Check sheet for the modelled part. Datum: model origin and axes. Units: mm. Give positions to 0.01 mm unless a question says otherwise; leave off trailing zeros. Order: outer loops, then holes, each group sorted by start corner. A loop starts at its lowest first (then second) coordinate and runs counter-clockwise, first axis right, second up. Notation, with made-up numbers: (-4.5, 52) -> (54.5, 52) arc R37 ccw to (54.5, 88) -> close; hole circle Ø3 at (-29, -38). An arc over 180 degrees is marked (long way). Write each question's results on one line, items separated by ' | '.
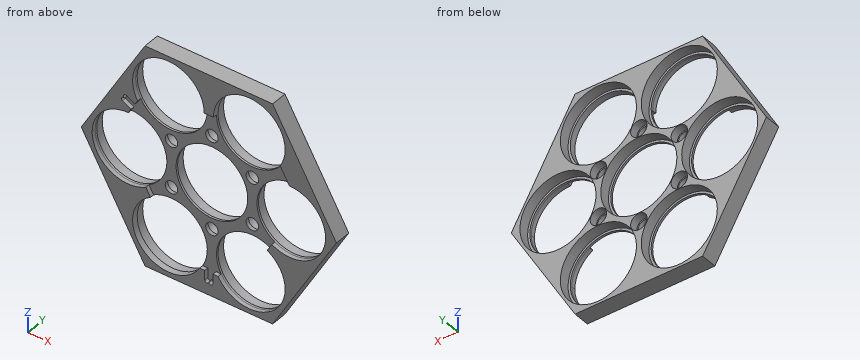
from build123d import *

# Parameters (mm, degrees)
SKETCH1_R                    = 17.5
BOSS_EXTRUDE1_DEPTH          = 1
SKETCH2_R                    = 18.575
BOSS_EXTRUDE2_DEPTH          = 5
CUT_EXTRUDE1_DEPTH           = 83.640310894
CUT_EXTRUDE1_DEPTH_BACK      = 4
SKETCH3_R                    = 4
SKETCH3_2_R                  = 4
CUT_EXTRUDE2_DEPTH           = 83.640310894
CUT_EXTRUDE2_DRAFT           = -9
CUT_EXTRUDE2_PROFILE_2_DEPTH = 83.640310894
CUT_EXTRUDE2_PROFILE_2_DRAFT = -9
CUT_EXTRUDE2_PROFILE_3_DEPTH = 83.640310894
CUT_EXTRUDE2_PROFILE_3_DRAFT = -9
CUT_EXTRUDE2_PROFILE_4_DEPTH = 83.640310894
CUT_EXTRUDE2_PROFILE_4_DRAFT = -9
CUT_EXTRUDE2_PROFILE_5_DEPTH = 83.640310894
CUT_EXTRUDE2_PROFILE_5_DRAFT = -9
CUT_EXTRUDE2_PROFILE_6_DEPTH = 83.640310894
CUT_EXTRUDE2_PROFILE_6_DRAFT = -9
BOSS_EXTRUDE3_START          = 2
BOSS_EXTRUDE3_DEPTH          = 2
CUT_EXTRUDE5_DEPTH           = 2


with BuildPart() as part:
    # Sketch1 → Boss-Extrude1 (new body)
    with BuildSketch(Plane(origin=(0, 0, 0), x_dir=(1, 0, 0), z_dir=(0, 1, 0))):
        Polygon((-31.152667816, -53.958003449), (31.152667816, -53.958003449), (62.305335633, 0), (31.152667816, 53.958003449), (-31.152667816, 53.958003449), (-62.305335633, 0), align=None)
        with Locations(Location((-39.5, 0, 0), (0, 0, 270))):
            Circle(SKETCH1_R, mode=Mode.SUBTRACT)
        with Locations(Location((-19.75, -34.208003449, 0), (0, 0, 270))):
            Circle(SKETCH1_R, mode=Mode.SUBTRACT)
        with Locations(Location((19.75, -34.208003449, 0), (0, 0, 270))):
            Circle(SKETCH1_R, mode=Mode.SUBTRACT)
        with Locations(Location((39.5, 0, 0), (0, 0, 270))):
            Circle(SKETCH1_R, mode=Mode.SUBTRACT)
        with Locations(Location((19.75, 34.208003449, 0), (0, 0, 270))):
            Circle(SKETCH1_R, mode=Mode.SUBTRACT)
        with Locations(Location((-19.75, 34.208003449, 0), (0, 0, 270))):
            Circle(SKETCH1_R, mode=Mode.SUBTRACT)
        with Locations(Location((0, 0, 0), (0, 0, 270))):
            Circle(SKETCH1_R, mode=Mode.SUBTRACT)
    extrude(amount=BOSS_EXTRUDE1_DEPTH)

    # Sketch2 → Boss-Extrude2 (add)
    with BuildSketch(Plane(origin=(0, 1, 0), x_dir=(1, 0, 0), z_dir=(0, 1, 0))):
        Polygon((62.305335633, 0), (31.152667816, 53.958003449), (-31.152667816, 53.958003449), (-62.305335633, 0), (-31.152667816, -53.958003449), (31.152667816, -53.958003449), align=None)
        with Locations(Location((-39.5, 0, 0), (0, 0, 270))):
            Circle(SKETCH2_R, mode=Mode.SUBTRACT)
        with Locations(Location((-19.75, 34.208003449, 0), (0, 0, 270))):
            Circle(SKETCH2_R, mode=Mode.SUBTRACT)
        with Locations(Location((19.75, 34.208003449, 0), (0, 0, 270))):
            Circle(SKETCH2_R, mode=Mode.SUBTRACT)
        with Locations(Location((0, 0, 0), (0, 0, 270))):
            Circle(SKETCH2_R, mode=Mode.SUBTRACT)
        with Locations(Location((39.5, 0, 0), (0, 0, 270))):
            Circle(SKETCH2_R, mode=Mode.SUBTRACT)
        with Locations(Location((19.75, -34.208003449, 0), (0, 0, 270))):
            Circle(SKETCH2_R, mode=Mode.SUBTRACT)
        with Locations(Location((-19.75, -34.208003449, 0), (0, 0, 270))):
            Circle(SKETCH2_R, mode=Mode.SUBTRACT)
    extrude(amount=BOSS_EXTRUDE2_DEPTH)

    # Sketch3 → Cut-Extrude1 (cut, two sides: drawn at the far end of the back side and taken through both)
    with BuildSketch(Plane(origin=(0, 6, 0), x_dir=(1, 0, 0), z_dir=(0, 1, 0)).offset(-CUT_EXTRUDE1_DEPTH_BACK)):
        with Locations(Location((-19.75, 11.402667816, 0), (0, 0, 90))):
            Circle(SKETCH3_R)
        with Locations(Location((19.75, 11.402667816, 0), (0, 0, 90))):
            Circle(SKETCH3_R)
        with Locations(Location((0, -22.805335633, 0), (0, 0, 90))):
            Circle(SKETCH3_R)
        with Locations(Location((-19.75, -11.402667816, 0), (0, 0, 90))):
            Circle(SKETCH3_R)
        with Locations(Location((19.75, -11.402667816, 0), (0, 0, 90))):
            Circle(SKETCH3_R)
        with Locations(Location((0, 22.805335633, 0), (0, 0, 90))):
            Circle(SKETCH3_R)
    extrude(amount=CUT_EXTRUDE1_DEPTH + CUT_EXTRUDE1_DEPTH_BACK, mode=Mode.SUBTRACT)


with BuildPart() as cut_extrude2_tool:
    # Sketch3<2> → Cut-Extrude2 (with draft: the straight prism first)
    with BuildSketch(Plane(origin=(0, 6, 0), x_dir=(1, 0, 0), z_dir=(0, 1, 0))):
        with Locations(Location((-19.75, 11.402667816, 0), (0, 0, 90))):
            Circle(SKETCH3_2_R)
    extrude(amount=-CUT_EXTRUDE2_DEPTH)
    # Cut-Extrude2: the draft: its side faces are tilted about the plane it starts from
    cut_extrude2_sides = [cut_extrude2_tool.faces().sort_by_distance(p)[0] for p in [
        (-19.75, -35.820155447, -7.402667816),
    ]]
    draft(cut_extrude2_sides, Plane(origin=(0, 6, 0), x_dir=(1, 0, 0), z_dir=(0, 1, 0)), CUT_EXTRUDE2_DRAFT)


with BuildPart() as part_1:
    add(part.part)

    # Cut-Extrude2: cut by cut_extrude2_tool
    add(cut_extrude2_tool.part, mode=Mode.SUBTRACT)


with BuildPart() as cut_extrude2_profile_2_tool:
    # Sketch3<2> → Cut-Extrude2 profile 2 (with draft: the straight prism first)
    with BuildSketch(Plane(origin=(0, 6, 0), x_dir=(1, 0, 0), z_dir=(0, 1, 0))):
        with Locations(Location((19.75, 11.402667816, 0), (0, 0, 90))):
            Circle(SKETCH3_2_R)
    extrude(amount=-CUT_EXTRUDE2_PROFILE_2_DEPTH)
    # Cut-Extrude2 profile 2: the draft: its side faces are tilted about the plane it starts from
    cut_extrude2_profile_2_sides = [cut_extrude2_profile_2_tool.faces().sort_by_distance(p)[0] for p in [
        (19.75, -35.820155447, -7.402667816),
    ]]
    draft(cut_extrude2_profile_2_sides, Plane(origin=(0, 6, 0), x_dir=(1, 0, 0), z_dir=(0, 1, 0)), CUT_EXTRUDE2_PROFILE_2_DRAFT)


with BuildPart() as part_2:
    add(part_1.part)

    # Cut-Extrude2 profile 2: cut by cut_extrude2_profile_2_tool
    add(cut_extrude2_profile_2_tool.part, mode=Mode.SUBTRACT)


with BuildPart() as cut_extrude2_profile_3_tool:
    # Sketch3<2> → Cut-Extrude2 profile 3 (with draft: the straight prism first)
    with BuildSketch(Plane(origin=(0, 6, 0), x_dir=(1, 0, 0), z_dir=(0, 1, 0))):
        with Locations(Location((0, -22.805335633, 0), (0, 0, 90))):
            Circle(SKETCH3_2_R)
    extrude(amount=-CUT_EXTRUDE2_PROFILE_3_DEPTH)
    # Cut-Extrude2 profile 3: the draft: its side faces are tilted about the plane it starts from
    cut_extrude2_profile_3_sides = [cut_extrude2_profile_3_tool.faces().sort_by_distance(p)[0] for p in [
        (0, -35.820155447, 26.805335633),
    ]]
    draft(cut_extrude2_profile_3_sides, Plane(origin=(0, 6, 0), x_dir=(1, 0, 0), z_dir=(0, 1, 0)), CUT_EXTRUDE2_PROFILE_3_DRAFT)


with BuildPart() as part_3:
    add(part_2.part)

    # Cut-Extrude2 profile 3: cut by cut_extrude2_profile_3_tool
    add(cut_extrude2_profile_3_tool.part, mode=Mode.SUBTRACT)


with BuildPart() as cut_extrude2_profile_4_tool:
    # Sketch3<2> → Cut-Extrude2 profile 4 (with draft: the straight prism first)
    with BuildSketch(Plane(origin=(0, 6, 0), x_dir=(1, 0, 0), z_dir=(0, 1, 0))):
        with Locations(Location((-19.75, -11.402667816, 0), (0, 0, 90))):
            Circle(SKETCH3_2_R)
    extrude(amount=-CUT_EXTRUDE2_PROFILE_4_DEPTH)
    # Cut-Extrude2 profile 4: the draft: its side faces are tilted about the plane it starts from
    cut_extrude2_profile_4_sides = [cut_extrude2_profile_4_tool.faces().sort_by_distance(p)[0] for p in [
        (-19.75, -35.820155447, 15.402667816),
    ]]
    draft(cut_extrude2_profile_4_sides, Plane(origin=(0, 6, 0), x_dir=(1, 0, 0), z_dir=(0, 1, 0)), CUT_EXTRUDE2_PROFILE_4_DRAFT)


with BuildPart() as part_4:
    add(part_3.part)

    # Cut-Extrude2 profile 4: cut by cut_extrude2_profile_4_tool
    add(cut_extrude2_profile_4_tool.part, mode=Mode.SUBTRACT)


with BuildPart() as cut_extrude2_profile_5_tool:
    # Sketch3<2> → Cut-Extrude2 profile 5 (with draft: the straight prism first)
    with BuildSketch(Plane(origin=(0, 6, 0), x_dir=(1, 0, 0), z_dir=(0, 1, 0))):
        with Locations(Location((19.75, -11.402667816, 0), (0, 0, 90))):
            Circle(SKETCH3_2_R)
    extrude(amount=-CUT_EXTRUDE2_PROFILE_5_DEPTH)
    # Cut-Extrude2 profile 5: the draft: its side faces are tilted about the plane it starts from
    cut_extrude2_profile_5_sides = [cut_extrude2_profile_5_tool.faces().sort_by_distance(p)[0] for p in [
        (19.75, -35.820155447, 15.402667816),
    ]]
    draft(cut_extrude2_profile_5_sides, Plane(origin=(0, 6, 0), x_dir=(1, 0, 0), z_dir=(0, 1, 0)), CUT_EXTRUDE2_PROFILE_5_DRAFT)


with BuildPart() as part_5:
    add(part_4.part)

    # Cut-Extrude2 profile 5: cut by cut_extrude2_profile_5_tool
    add(cut_extrude2_profile_5_tool.part, mode=Mode.SUBTRACT)


with BuildPart() as cut_extrude2_profile_6_tool:
    # Sketch3<2> → Cut-Extrude2 profile 6 (with draft: the straight prism first)
    with BuildSketch(Plane(origin=(0, 6, 0), x_dir=(1, 0, 0), z_dir=(0, 1, 0))):
        with Locations(Location((0, 22.805335633, 0), (0, 0, 90))):
            Circle(SKETCH3_2_R)
    extrude(amount=-CUT_EXTRUDE2_PROFILE_6_DEPTH)
    # Cut-Extrude2 profile 6: the draft: its side faces are tilted about the plane it starts from
    cut_extrude2_profile_6_sides = [cut_extrude2_profile_6_tool.faces().sort_by_distance(p)[0] for p in [
        (0, -35.820155447, -18.805335633),
    ]]
    draft(cut_extrude2_profile_6_sides, Plane(origin=(0, 6, 0), x_dir=(1, 0, 0), z_dir=(0, 1, 0)), CUT_EXTRUDE2_PROFILE_6_DRAFT)


with BuildPart() as part_6:
    add(part_5.part)

    # Cut-Extrude2 profile 6: cut by cut_extrude2_profile_6_tool
    add(cut_extrude2_profile_6_tool.part, mode=Mode.SUBTRACT)

    # Sketch5 → Boss-Extrude3 (add)
    with BuildSketch(Plane.XZ.offset(BOSS_EXTRUDE3_START)):
        with BuildLine():
            Line((-31.152667816, 53.958003449), (-62.305335633, 0))
            Line((-62.305335633, 0), (-57, 0))
            ThreePointArc((-57, 0), (-51.812065653, 12.43635957), (-39.324224074, 17.499117201))
            Line((-39.324224074, 17.499117201), (-34.816792077, 25.306218432))
            ThreePointArc((-34.816792077, 25.306218432), (-24.364170491, 51.088744863), (-2.25, 34.208003449))
            Line((-2.25, 34.208003449), (2.25, 34.208003449))
            ThreePointArc((2.25, 34.208003449), (11, 49.363448016), (28.5, 49.363448016))
            Line((28.5, 49.363448016), (31.152667816, 53.958003449))
            Line((31.152667816, 53.958003449), (-31.152667816, 53.958003449))
        make_face()
        with BuildLine():
            Line((-57, 0), (-62.305335633, 0))
            Line((-62.305335633, 0), (-31.152667816, -53.958003449))
            Line((-31.152667816, -53.958003449), (31.152667816, -53.958003449))
            Line((31.152667816, -53.958003449), (28.5, -49.363448016))
            ThreePointArc((28.5, -49.363448016), (15.135829509, -51.088744863), (4.507431997, -42.805335633))
            Line((4.507431997, -42.805335633), (-4.507431997, -42.805335633))
            ThreePointArc((-4.507431997, -42.805335633), (-32.062065653, -46.644363019), (-28.5, -19.052558883))
            Line((-28.5, -19.052558883), (-30.75, -15.155444566))
            ThreePointArc((-30.75, -15.155444566), (-48.25, -15.155444566), (-57, 0))
        make_face()
        with BuildLine():
            Line((28.5, -49.363448016), (31.152667816, -53.958003449))
            Line((31.152667816, -53.958003449), (62.305335633, 0))
            Line((62.305335633, 0), (31.152667816, 53.958003449))
            Line((31.152667816, 53.958003449), (28.5, 49.363448016))
            ThreePointArc((28.5, 49.363448016), (34.905444566, 42.958003449), (37.25, 34.208003449))
            ThreePointArc((37.25, 34.208003449), (36.630741414, 29.593832958), (34.816792077, 25.306218432))
            Line((34.816792077, 25.306218432), (39.324224074, 17.499117201))
            ThreePointArc((39.324224074, 17.499117201), (51.812065653, 12.43635957), (57, 0))
            ThreePointArc((57, 0), (48.25, -15.155444566), (30.75, -15.155444566))
            Line((30.75, -15.155444566), (28.5, -19.052558883))
            ThreePointArc((28.5, -19.052558883), (34.905444566, -25.458003449), (37.25, -34.208003449))
            ThreePointArc((37.25, -34.208003449), (34.905444566, -42.958003449), (28.5, -49.363448016))
        make_face()
    extrude(amount=-BOSS_EXTRUDE3_DEPTH)

    # Sketch6 → Cut-Extrude5 (cut)
    with BuildSketch(Plane.XZ.offset(2)):
        with BuildLine():
            ThreePointArc((-2, -47.537386441), (-1, -48.537386441), (0, -47.537386441))
            ThreePointArc((0, -47.537386441), (1, -48.537386441), (2, -47.537386441))
            Line((2, -47.537386441), (2, -42.805335633))
            Line((2, -42.805335633), (-2, -42.805335633))
            Line((-2, -42.805335633), (-2, -47.537386441))
        make_face()
        with BuildLine():
            ThreePointArc((-40.168584287, 25.500744028), (-41.534609686, 25.134718633), (-41.168584305, 23.76869323))
            ThreePointArc((-41.168584305, 23.76869323), (-42.534609696, 23.402667808), (-42.168584287, 22.036642413))
            Line((-42.168584287, 22.036642413), (-38.070508076, 19.670617009))
            Line((-38.070508076, 19.670617009), (-36.070508076, 23.134718624))
            Line((-36.070508076, 23.134718624), (-40.168584287, 25.500744028))
        make_face()
    extrude(amount=-CUT_EXTRUDE5_DEPTH, mode=Mode.SUBTRACT)


solid = part_6.part
1. Section check C-C on x = -14. Record the cut outline in (y, z), then the cut area to 3 significant figures.
Verdict:
outline: (-2, -53.96) -> (6, -53.96) -> (6, -51.87) -> (1, -51.87) -> (1, -50.74) -> (-2, -50.74) -> close; (-2, 50.74) -> (1, 50.74) -> (1, 51.87) -> (6, 51.87) -> (6, 53.96) -> (-2, 53.96) -> close; (0, -17.68) -> (1, -17.68) -> (1, -16.55) -> (6, -16.55) -> (6, -12.21) -> (1, -12.21) -> (1, -10.5) -> (0, -10.5) -> close; (0, 10.5) -> (1, 10.5) -> (1, 12.21) -> (6, 12.21) -> (6, 16.55) -> (1, 16.55) -> (1, 17.68) -> (0, 17.68) -> close | area: 97.9 mm^2
2. Section check B-B on z = -30. Record the cut outline in (x, y).
Verdict:
outline: (-44.98, -2) -> (-36.74, -2) -> (-36.74, 1) -> (-37.84, 1) -> (-37.84, 6) -> (-44.98, 6) -> close; (-2.76, 0) -> (2.76, 0) -> (2.76, 1) -> (1.66, 1) -> (1.66, 6) -> (-1.66, 6) -> (-1.66, 1) -> (-2.76, 1) -> close; (36.74, -2) -> (44.98, -2) -> (44.98, 6) -> (37.84, 6) -> (37.84, 1) -> (36.74, 1) -> close
3. Material ranges on probe 1 along X at (y, z) = (0.7, 0); probe 2 along X at (y, z) = (5, 0) (3 decimals); probe 3 along X at (y, z) = (2.5, 31), recorded low to high. Write a range as from..to.
Verdict:
probe 1: x = -62.31..-57, -22..-17.5, 17.5..22, 57..62.31 | probe 2: x = -62.305..-58.075, -20.925..-18.575, 18.575..20.925, 58.075..62.305 | probe 3: x = -44.41..-38.05, -1.45..1.45, 38.05..44.41
4. Section check A-A on y = 4.75. Give the number of separate pieces and of enclosed holes in the cut face, then the cut area to 3 significant figures.
Verdict:
separate pieces: 1 | enclosed holes: 13 | area: 2,200 mm^2
5. Gauge pin test, flat ends, axial feed: pin 1 Ø1.5 at (y, z) = (4.5, -12) entering from -X; pin 2 Ø21 at (x, z) = (19.75, 34.21) entering from -Y; pin 3 Ø10.5 at (x, z) = (0, 22.81) entering from -Y; pin 4 Ø2 at (y, z) = (0.5, 2.5) entering from -X. Record the tip position at first contact, or that the pin passes through.
Verdict:
pin 1: stops at x = -55.81 | pin 2: passes through | pin 3: stops at y = 0 | pin 4: stops at x = -61.44
